```python
from build123d import *

# Parameters (mm, degrees)
SKETCH_1_R          = 30
SKETCH_1_R_2        = 26.5
EXTRUDE_1_DEPTH     = 15
SKETCH_2_R          = 30
EXTRUDE_2_DEPTH     = 2
CHAMFER_1_SIZE      = 5
SKETCH_3_R          = 1.65
CUT_EXTRUDE_1_DEPTH = 44.957365708


with BuildPart() as part:
    # 草图1 → 凸台-拉伸1 (new body)
    with BuildSketch(Plane(origin=(0, 0, 0), x_dir=(1, 0, 0), z_dir=(0, 1, 0))):
        with Locations(Location((0, 0, 0), (0, 0, 270))):
            Circle(SKETCH_1_R)
        with Locations(Location((0, 0, 0), (0, 0, 270))):
            Circle(SKETCH_1_R_2, mode=Mode.SUBTRACT)
    extrude(amount=EXTRUDE_1_DEPTH)

    # 草图2 → 凸台-拉伸2 (add)
    with BuildSketch(Plane.XZ):
        with Locations(Location((0, 0, 0), (0, 0, 90))):
            Circle(SKETCH_2_R)
    extrude(amount=-EXTRUDE_2_DEPTH)

    # 倒角1
    # the kernel refuses this chamfer: 5 mm, written as the material it takes off along each edge
    with BuildSketch(Plane(origin=(0, 15, 0), x_dir=(0, 0, 1), z_dir=(-1, 0, 0))) as chamfer_1_piece_1:
        Polygon((26.5 + CHAMFER_1_SIZE, 0), (26.5, -CHAMFER_1_SIZE), (26.5, 0), align=None)
    revolve(axis=Axis((0, 15, 0), (0, 1, 0)), mode=Mode.SUBTRACT)

    # 草图3 → 切除-拉伸1 (cut, through all)
    with BuildSketch(Plane(origin=(0, 2, 0), x_dir=(1, 0, 0), z_dir=(0, 1, 0))):
        with Locations(Location((0, 0, 0), (0, 0, 270))):
            Circle(SKETCH_3_R)
    extrude(amount=-CUT_EXTRUDE_1_DEPTH, mode=Mode.SUBTRACT)


solid = part.part
```
Could you check a few things on this model? Use its own coordinates, in mm. Give positions to 0.01 mm unless a question says otherwise; leave off trailing zeros. Loops run counter-clockwise (first coordinate to the right, second up) from the corner with the lowest first, then second, coordinate; pieces in that order, holes last. Notation, with made-up numbers: (45.25, 20) - (73.25, 20) arc R30 ccw to (73.25, 52) - close; hole circle Ø2 at (37, 3.5). An arc over 180 degrees is marked (long way). Answer in a Markdown table with one row per item. Add a question column.
Q1. Please list where these lines run through material, in increasing order: L1, parallel to X at y = 6.25, z = 0; L2, parallel to X at y = 1.5, z = 0; L3, parallel to Y at x = 5, z = 8. Write a range as from..to.
Q2. If we section it at C-C (y = 8.75): List the corners of the cut face in (x, z) for me.
Q3. For pin 1 (3 mm diameter, centred on y = 2, z = 12, fed in from +X); pin 2 (1.5 mm diameter, centred on x = 3, y = 11.5, fed in from +Z); pin 3 (8 mm diameter, centred on y = 2.5, z = 8, fed in from +X); pin 4 (6 mm diameter, centred on x = -1.5, z = 21.5, fed in from -Y), each with a flat end and sliding along its axis, tell me the tip position at first contact or that it passes through.
Q4. We'd pull the mould along Z, two halves only. Please class faces 1 (the face through (-1, 1.01, -1.31)), 2 (the face through (1.32, 6.66, -29.97)), 3 (the face through (0, 0, 6)): +Z half, -Z half, draft (parallel to the pull), parting line (faces both ways), or undercut.
Q5. If we section it at B-B (z = 0): List the corners of the cut face in (x, y) for me.
Q6. If we section it at A-A (x = 0): List the corners of the cut face in (y, z) for me.
The answers:
| question | item | result |
|---|---|---|
| 1 | L1 | x = -30..-26.5, 26.5..30 |
| 1 | L2 | x = -30..-1.65, 1.65..30 |
| 1 | L3 | y = 0..2 |
| 2 | outline | circle Ø60 at (0, 0); hole circle Ø53 at (0, 0) |
| 3 | pin 1 | stops at x = 28.1 |
| 3 | pin 2 | stops at z = 29.92 |
| 3 | pin 3 | stops at x = 29.73 |
| 3 | pin 4 | stops at y = 0 |
| 4 | face 1 | undercut |
| 4 | face 2 | parting line |
| 4 | face 3 | draft |
| 5 | outline | (-30, 0) - (-1.65, 0) - (-1.65, 2) - (-26.5, 2) - (-26.5, 10) - (-30, 13.5) - close; (1.65, 0) - (30, 0) - (30, 13.5) - (26.5, 10) - (26.5, 2) - (1.65, 2) - close |
| 6 | outline | (0, -30) - (13.5, -30) - (10, -26.5) - (2, -26.5) - (2, -1.65) - (0, -1.65) - close; (0, 1.65) - (2, 1.65) - (2, 26.5) - (10, 26.5) - (13.5, 30) - (0, 30) - close |
